Job drawing, mm, ordinate dimensions from the low corner. One solid piece. A direction names the side the tool comes from. Round coordinates to 2 decimals unless told otherwise and drop trailing zeros. Loops run counter-clockwise (first coordinate to the right, second up) from the corner with the lowest first, then second, coordinate; pieces in that order, holes last.
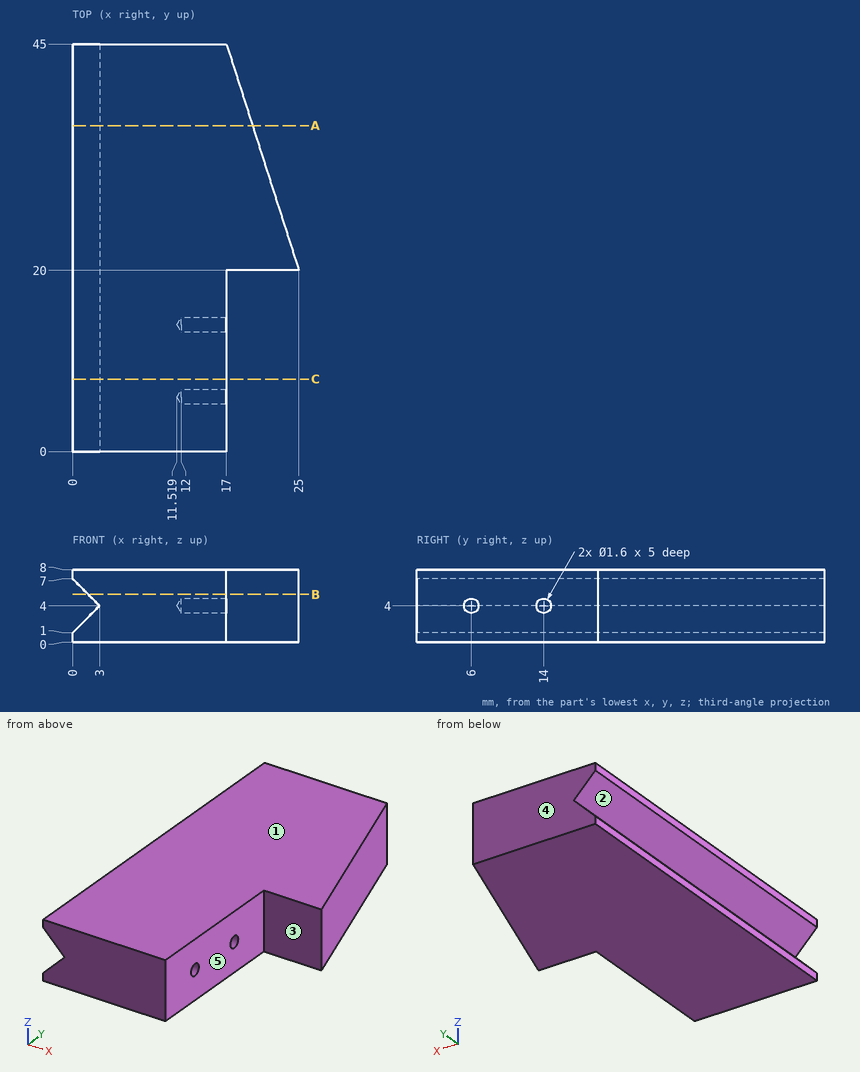
(1) Pin check, flat tips, straight feed: P1, Ø1, axis at x = 19, y = 14.5, coming from the +Z side; P2, Ø3, axis at x = 18, z = 2, coming from the -Y side; P3, Ø3, axis at y = 7.5, z = 3, coming from the +X side; P4, Ø1, axis at y = 14, z = 4, coming from the -X side. Stop position of each tip, or through.
Responses:
P1: passes through
P2: stops at y = 0
P3: stops at x = 17
P4: stops at x = 2.5
(2) Which spindle directions (+Z, -Z, +X, -X, +Y, -Y) get a long thin tool onto all of the face, cutting with end or side? Do the marked faces 4 and 5. Say none if no direction does.
Responses:
face 4: +Z, -Z, +X, -X, +Y
face 5: +Z, -Z, +X, -Y
(3) Slice it at B-B on z = 5.25. List the corners of the cut face in (x, y), plus the area to 3 significant figures.
Responses:
outline: (1.75, 0) - (17, 0) - (17, 20) - (25, 20) - (17, 45) - (1.75, 45) - close
area: 786 mm2
(4) Probe line 1 (Y direction, x = 14, z = 4); line 2 (Y direction, x = 16.25, z = 3.5) (1 decimal); line 3 (X direction, y = 9.5, z = 2). List the from-to ranges inside material, lowest first.
Responses:
line 1: y = 0 to 5.2, 6.8 to 13.2, 14.8 to 45
line 2: y = 0 to 5.4, 6.6 to 13.4, 14.6 to 45
line 3: x = 1 to 17
(5) Slice it at A-A on y = 36. List the corners of the cut face in (x, z), plus the area to 3 significant figures.
Responses:
outline: (0, 0) - (19.88, 0) - (19.88, 8) - (0, 8) - (0, 7) - (3, 4) - (0, 1) - close
area: 150 mm2
(6) Slice it at C-C on y = 8. List the corners of the cut face in (x, z), plus the area to 3 significant figures.
Responses:
outline: (0, 0) - (17, 0) - (17, 8) - (0, 8) - (0, 7) - (3, 4) - (0, 1) - close
area: 127 mm2
(7) Pull direction Z, two halves, no side cores. Call the marked faces 1, 2 and 3: +Z half, -Z half, draft (parallel to the pull), parting line (faces both ways), or undercut.
Responses:
face 1: +Z half
face 2: undercut
face 3: draft
